CAD build for the part. Positions are in the model's coordinates, mm. Face numbers are marked on the shaded views. A direction names the side the tool comes from. Give positions to 0.01 mm unless a question says otherwise; leave off trailing zeros. Write each loop counter-clockwise with the first axis right and the second up, starting at its lowest first coordinate (ties: lowest second). Pieces come first, ordered by that corner, then holes. Notation, with made-up numbers: (3.5, 23) -> (62.5, 23) arc R16 ccw to (62.5, 51) -> close; hole circle Ø7 at (-8, 39.25). An arc over 180 degrees is marked (long way). Answer as a JSON object with one key per item and string values.
```python
from build123d import *

# Parameters (mm, degrees)
BOSS_EXTRUDE1_DEPTH = 6.35


with BuildPart() as part:
    # Sketch2 → Boss-Extrude1 (new body)
    with BuildSketch(Plane(origin=(0, 0, 0), x_dir=(0, 0, -1), z_dir=(1, 0, 0))):
        with BuildLine():
            Line((14.859, 42.418), (14.859, 55.118))
            Line((14.859, 55.118), (8.509, 55.118))
            Line((8.509, 55.118), (8.509, 36.068))
            Line((8.509, 36.068), (0, 36.068))
            Line((0, 36.068), (0, 5.08))
            ThreePointArc((0, 5.08), (1.487897552, 1.487897552), (5.08, 0))
            Line((5.08, 0), (14.859, 0))
            Line((14.859, 0), (14.859, 6.35))
            Line((14.859, 6.35), (11.43, 6.35))
            ThreePointArc((11.43, 6.35), (7.837897552, 7.837897552), (6.35, 11.43))
            Line((6.35, 11.43), (6.35, 24.638))
            ThreePointArc((6.35, 24.638), (7.837897552, 28.230102448), (11.43, 29.718))
            Line((11.43, 29.718), (14.859, 29.718))
            Line((14.859, 29.718), (14.859, 36.068))
            Line((14.859, 36.068), (21.209, 36.068))
            Line((21.209, 36.068), (21.209, 29.718))
            Line((21.209, 29.718), (24.638, 29.718))
            ThreePointArc((24.638, 29.718), (28.230102448, 28.230102448), (29.718, 24.638))
            Line((29.718, 24.638), (29.718, 11.43))
            ThreePointArc((29.718, 11.43), (28.230102448, 7.837897552), (24.638, 6.35))
            Line((24.638, 6.35), (21.209, 6.35))
            Line((21.209, 6.35), (21.209, 0))
            Line((21.209, 0), (30.988, 0))
            ThreePointArc((30.988, 0), (34.580102448, 1.487897552), (36.068, 5.08))
            Line((36.068, 5.08), (36.068, 36.068))
            Line((36.068, 36.068), (27.559, 36.068))
            Line((27.559, 36.068), (27.559, 55.118))
            Line((27.559, 55.118), (21.209, 55.118))
            Line((21.209, 55.118), (21.209, 42.418))
            Line((21.209, 42.418), (14.859, 42.418))
        make_face()
    extrude(amount=BOSS_EXTRUDE1_DEPTH)


solid = part.part
```
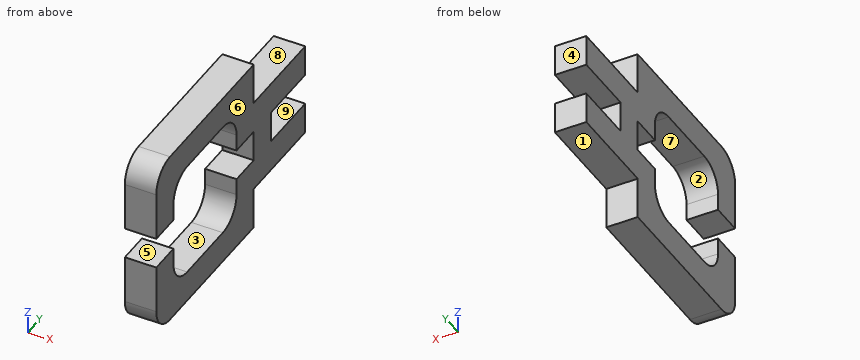
1) Wall check: probe 1 along Y at (x, z) = (5, -23); probe 2 along Z at (x, y) = (1, 15.5); probe 3 along Z at (x, y) = (5.75, 46). Give the ranges that are in metal, low to high.
Model answer:
{"probe 1": "y = 0 to 6.35, 29.72 to 55.12", "probe 2": "z = -36.07 to -29.72, -6.35 to 0", "probe 3": "z = -27.56 to -21.21, -14.86 to -8.51"}
2) Slice it at A-A (y = 35). List the corners of the cut face in (x, z), then the cut area to 3 significant figures.
Model answer:
{"outline": "(0, -36.07) -> (6.35, -36.07) -> (6.35, -21.21) -> (0, -21.21) -> close; (0, -14.86) -> (6.35, -14.86) -> (6.35, 0) -> (0, 0) -> close", "area": "189 mm2"}
3) Mould opens along Z. For the marked faces 1, 2, 3 and 4 say: released by +Z, released by -Z, zero draft, split by the parting line, or undercut.
Model answer:
{"face 1": "released by -Z", "face 2": "undercut", "face 3": "undercut", "face 4": "zero draft"}
4) 3-axis set-ups, long thin cutter, end or side, ignore diameter. For the marked faces 5, 6, 7, 8 and 9: which of +Z, -Z, +X, -X, +Y, -Y reach the whole face in a straight line?
Model answer:
{"face 5": "+X, -X, -Y", "face 6": "+Z, -Z, +X, +Y, -Y", "face 7": "+X, -X", "face 8": "+Z, +X, -X, +Y", "face 9": "+X, -X, +Y"}
5) Slice it at B-B (z = -12). List the corners of the cut face in (x, y), then the cut area to 3 significant figures.
Model answer:
{"outline": "(0, 0) -> (6.35, 0) -> (6.35, 6.35) -> (0, 6.35) -> close; (0, 29.72) -> (6.35, 29.72) -> (6.35, 55.12) -> (0, 55.12) -> close", "area": "202 mm2"}
6) Slice it at D-D (z = -16). List the corners of the cut face in (x, y).
Model answer:
{"outline": "(0, 36.07) -> (6.35, 36.07) -> (6.35, 42.42) -> (0, 42.42) -> close"}
7) Pin check, flat tips, straight feed: pin 1 (1.9 mm diameter, centred on x = 4, y = 48, fed in from +Z); pin 2 (3 mm diameter, centred on x = 3.5, y = 3, fed in from -Z); pin 3 (4 mm diameter, centred on y = 15, z = -27.5, fed in from +X); pin 4 (1.9 mm diameter, centred on x = 3.5, z = -16.5, fed in from -Y). Stop position of each tip, or through.
Model answer:
{"pin 1": "stops at z = -8.51", "pin 2": "stops at z = -36.03", "pin 3": "passes through", "pin 4": "stops at y = 36.07"}
